For this review, take the finished solid that the model builds, in its own axes (mm). A direction names the side the tool comes from. Round coordinates to 2 decimals unless told otherwise and drop trailing zeros. Write each loop counter-clockwise with the first axis right and the second up, starting at its lowest first coordinate (ties: lowest second). Pieces come first, ordered by that corner, then holes.
from build123d import *

# Parameters (mm, degrees)
SKETCH1_R           = 1.4
SKETCH1_R_2         = 2
BOSS_EXTRUDE1_DEPTH = 8
SKETCH2_R           = 3.75
BOSS_EXTRUDE2_DEPTH = 2
SKETCH3_R           = 3
BOSS_EXTRUDE3_DEPTH = 3
SKETCH4_R           = 1.4
CUT_EXTRUDE1_DEPTH  = 53.621288468
SKETCH5_R           = 5
CUT_EXTRUDE2_DEPTH  = 6
SKETCH6_R           = 5.25
CUT_EXTRUDE3_DEPTH  = 3.2
SKETCH7_R           = 5
CUT_EXTRUDE4_DEPTH  = 2
SKETCH8_R           = 4
CUT_EXTRUDE5_DEPTH  = 1
CUT_EXTRUDE6_DEPTH  = 52.613951602
FILLET1_R           = 2


with BuildPart() as part:
    # Sketch1 → Boss-Extrude1 (new body)
    with BuildSketch(Plane(origin=(0, 0, 0), x_dir=(1, 0, 0), z_dir=(0, 1, 0))):
        with BuildLine():
            Line((-40, -10), (40, -10))
            ThreePointArc((40, -10), (50, 0), (40, 10))
            Line((40, 10), (-40, 10))
            ThreePointArc((-40, 10), (-50, 0), (-40, -10))
        make_face()
        with Locations(Location((-40, 0, 0), (0, 0, 270))):
            Circle(SKETCH1_R, mode=Mode.SUBTRACT)
        with Locations(Location((40, 0, 0), (0, 0, 270))):
            Circle(SKETCH1_R_2, mode=Mode.SUBTRACT)
    extrude(amount=BOSS_EXTRUDE1_DEPTH)

    # Sketch2 → Boss-Extrude2 (add)
    with BuildSketch(Plane(origin=(0, 8, 0), x_dir=(1, 0, 0), z_dir=(0, 1, 0))):
        with Locations(Location((-40, 0, 0), (0, 0, 90))):
            Circle(SKETCH2_R)
    extrude(amount=BOSS_EXTRUDE2_DEPTH)

    # Sketch3 → Boss-Extrude3 (add)
    with BuildSketch(Plane(origin=(0, 10, 0), x_dir=(1, 0, 0), z_dir=(0, 1, 0))):
        with Locations(Location((-40, 0, 0), (0, 0, 270))):
            Circle(SKETCH3_R)
    extrude(amount=BOSS_EXTRUDE3_DEPTH)

    # Sketch4 → Cut-Extrude1 (cut, through all)
    with BuildSketch(Plane.XZ):
        with Locations(Location((-40, 0, 0), (0, 0, 270))):
            Circle(SKETCH4_R)
    extrude(amount=-CUT_EXTRUDE1_DEPTH, mode=Mode.SUBTRACT)

    # Sketch5 → Cut-Extrude2 (cut)
    with BuildSketch(Plane.XZ):
        with Locations(Location((-40, 0, 0), (0, 0, 270))):
            Circle(SKETCH5_R)
    extrude(amount=-CUT_EXTRUDE2_DEPTH, mode=Mode.SUBTRACT)

    # Sketch6 → Cut-Extrude3 (cut)
    with BuildSketch(Plane.XZ):
        with Locations(Location((40, 0, 0), (0, 0, 270))):
            Circle(SKETCH6_R)
    extrude(amount=-CUT_EXTRUDE3_DEPTH, mode=Mode.SUBTRACT)

    # Sketch7 → Cut-Extrude4 (cut)
    with BuildSketch(Plane(origin=(0, 8, 0), x_dir=(1, 0, 0), z_dir=(0, 1, 0))):
        with Locations(Location((40, 0, 0), (0, 0, 270))):
            Circle(SKETCH7_R)
    extrude(amount=-CUT_EXTRUDE4_DEPTH, mode=Mode.SUBTRACT)

    # Sketch8 → Cut-Extrude5 (cut)
    with BuildSketch(Plane.XZ.offset(-3.2)):
        with Locations(Location((40, 0, 0), (0, 0, 270))):
            Circle(SKETCH8_R)
    extrude(amount=-CUT_EXTRUDE5_DEPTH, mode=Mode.SUBTRACT)

    # Sketch9 → Cut-Extrude6 (cut, symmetric)
    with BuildSketch(Plane(origin=(0, 8, 0), x_dir=(1, 0, 0), z_dir=(0, 1, 0))):
        with BuildLine():
            Line((-40, 10), (40, 10))
            ThreePointArc((40, 10), (0, 7.994974843), (-40, 10))
        make_face()
    cut_extrude6 = extrude(amount=CUT_EXTRUDE6_DEPTH, both=True, mode=Mode.SUBTRACT)

    # Mirror1: Cut-Extrude6 across plane
    add(cut_extrude6.mirror(Plane.XY), mode=Mode.SUBTRACT)

    # Fillet1
    fillet1_edges = [part.edges().sort_by_distance(p)[0] for p in [
        (-40, 4, 10),
        (-40, 4, -10),
    ]]
    fillet(fillet1_edges, radius=FILLET1_R)


solid = part.part
(1) We need section A-A, the plane y = 1.75. State how many separate pieces and enclosed holes the cut face has, and give its area (3 significant figures).
Geometry check:
separate pieces: 1
enclosed holes: 2
area: 1,540 mm2
(2) We need section D-D, the plane x = -10. Give the boundary of the cut face in (y, z).
Geometry check:
outline: (0, -8.12) - (8, -8.12) - (8, 8.12) - (0, 8.12) - close
(3) For faces 1 (the face through (-37.47, 11.48, 1.61)), 2 (the face through (0.613, 4.056, -7.995)), 3 (the face through (43.966, 3.693, 0.521)), list the 3-axis set-ups (+Z, -Z, +X, -X, +Y, -Y) from which the entire face can be reached by the end or side of a thin tool; tool diameter is ignored.
Geometry check:
face 1: +Y
face 2: -Z, +Y, -Y
face 3: -Y
(4) Mouldability with a two-part tool opening along Z and no side actions: class faces 4 (the face through (38, 5, 0)), 5 (the face through (50, 4, 0)), 6 (the face through (-1, 0, 0)), 7 (the face through (44.957, 7.014, -0.651)) as pulls with the +Z half, pulls with the -Z half, needs draft (parallel to the pull), parting line crosses it, or undercut.
Geometry check:
face 4: undercut
face 5: parting line crosses it
face 6: needs draft
face 7: undercut
(5) We need section C-C, the plane y = 11. Give the boundary of the cut face in (x, z).
Geometry check:
outline: circle Ø6 at (-40, 0); hole circle Ø2.8 at (-40, 0)
(6) For pin 1 Ø1.5 at (y, z) = (5, 0.5) entering from -X; pin 2 Ø9 at (x, z) = (40, 0) entering from -Y; pin 3 Ø10 at (x, z) = (-31.5, 6.5) entering from +Y; pin 4 Ø5 at (y, z) = (9, -6) entering from +X, all flat-tipped, find the tip position at first contact; note any pin that passes through.
Geometry check:
pin 1: stops at x = -50
pin 2: stops at y = 3.2
pin 3: stops at y = 8
pin 4: stops at x = 49.29
(7) For line 1 along X through (y, z) = (2.3, 0); line 2 along X through (y, z) = (6.7, 0); line 3 along Y through (x, z) = (-43, -3.5), list the stretches that pass through material, from the lowest coordinate up.
Geometry check:
line 1: x = -50 to -45, -35 to 34.75, 45.25 to 50
line 2: x = -50 to -41.4, -38.6 to 35, 45 to 50
line 3: y = 6 to 8
